```python
from build123d import *

# Parameters (mm, degrees)
F0_R     = 15
F1_DEPTH = 15
F2_R     = 15
F3_DEPTH = 10
F4_R     = 30
F4_R_2   = 15
F5_DEPTH = 10


with BuildPart() as f1:
    # F0 (on Front) → F1 (new body)
    with BuildSketch(Plane.XZ):
        with BuildLine():
            ThreePointArc((30, 15), (27.071068, 22.071068), (20, 25))
            Line((20, 25), (-20, 25))
            ThreePointArc((-20, 25), (-27.071068, 22.071068), (-30, 15))
            Line((-30, 15), (-30, -25))
            Line((-30, -25), (30, -25))
            Line((30, -25), (30, 15))
        make_face()
        with Locations((0, 5)):
            Circle(F0_R, mode=Mode.SUBTRACT)
    extrude(amount=F1_DEPTH)

    # F2 (on face) → F3 (join)
    with BuildSketch(Plane(origin=(0, 0, -25), x_dir=(1, 0, 0), z_dir=(0, 0, -1))):
        with BuildLine():
            ThreePointArc((11.14172, 62.145699), (24.842017, 73.181136), (30, 90))
            ThreePointArc((30, 90), (0, 120), (-30, 90))
            ThreePointArc((-30, 90), (-16.818864, 65.157983), (11.14172, 62.145699))
        make_face()
        with Locations((0, 90)):
            Circle(F2_R, mode=Mode.SUBTRACT)
        with BuildLine():
            ThreePointArc((11.14172, 62.145699), (-16.818864, 65.157983), (-30, 90))
            Line((-30, 90), (-30, 15))
            Line((-30, 15), (-30, 0))
            Line((-30, 0), (30, 0))
            Line((30, 0), (30, 15))
            Line((30, 15), (11.14172, 62.145699))
        make_face()
    extrude(amount=F3_DEPTH)

    # F4 (on face) → F5 (join)
    with BuildSketch(Plane(origin=(0, 0, -35), x_dir=(1, 0, 0), z_dir=(0, 0, -1))):
        with Locations((0, 90)):
            Circle(F4_R)
        with Locations((0, 90)):
            Circle(F4_R_2, mode=Mode.SUBTRACT)
    extrude(amount=F5_DEPTH)


solid = f1.part
```
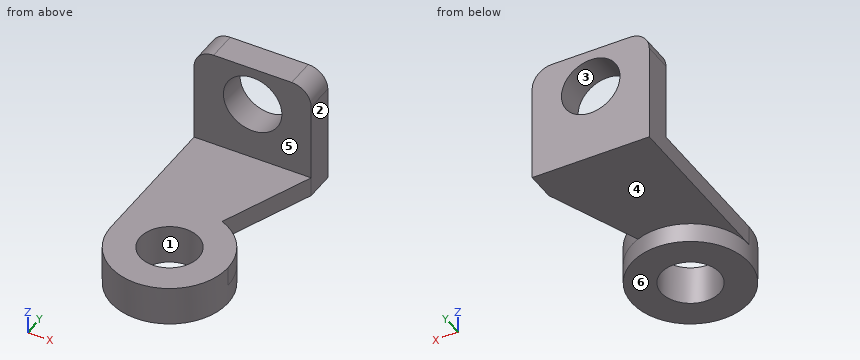
Part model, mm, in its own coordinate system. Face numbers are marked on the shaded views. A direction names the side the tool comes from. Round coordinates to 2 decimals unless told otherwise and drop trailing zeros. Order: outer loops, then holes, each group sorted by start corner. A loop starts at its lowest first (then second) coordinate and runs counter-clockwise, first axis right, second up. Notation, with made-up numbers: M 27.25,79 L 31.25,79 A19 cw 31.25,91 Z; hole C 70.25,62.25 d2. An arc over 180 degrees is marked long. Put each result on its own line as item: value. Start each with the question number.
1. Two-plate mould, pull along X, no slides. Class the marked faces 1, 2, 3 and 4: +X half, -X half, draft (parallel to the pull), parting line (faces both ways), or undercut.
2. Tool access for the marked faces 5 and 6: list every direction of +Z, -Z, +X, -X, +Y, -Y with a clear straight run to the whole face (end or side of a thin tool).
3. Slice it at B-B on z = 17. List the corners of the cut face in (x, y), then the cut area to 3 significant figures.
4. Slice it at D-D on z = -33. List the corners of the cut face in (x, y), then the cut area to 3 significant figures.
5. Drop flat-ended pins along their axis: pin 1 (10 mm diameter, centred on x = -9.5, z = 14.5, fed in from -Y); pin 2 (2 mm diameter, centred on x = 4.5, y = -34, fed in from -Z); pin 3 (5 mm diameter, centred on x = 18, y = -29, fed in from +Z). Give the stop position or say it passes through.
6. Drill centre lines: probe 1 along Z at (x, y) = (0, -4.5); probe 2 along X at (y, z) = (-90, -32); probe 3 along Z at (x, y) = (-6, -65). Where is each one in solid material? Low to high. Write a range as [from, to].
7. Slice it at C-C on y = -84. List the corners of the cut face in (x, z), then the cut area to 3 significant figures.
8. Slice it at A-A on x = 0. List the corners of the cut face in (y, z).
Findings:
1. face 1: undercut
1. face 2: +X half
1. face 3: undercut
1. face 4: draft
2. face 5: +Z, +X, -X, -Y
2. face 6: -Z, +X, -X, +Y, -Y
3. outline: M -29.8,-15 L -9,-15 L -9,0 L -29.8,0 Z; M 9,-15 L 29.8,-15 L 29.8,0 L 9,0 Z
3. area: 624 mm2
4. outline: M -30,-90 A30 ccw long 11.14,-62.15 L 30,-15 L 30,0 L -30,0 Z; hole C 0,-90 d30
4. area: 5,520 mm2
5. pin 1: y = -15
5. pin 2: z = -35
5. pin 3: z = -25
6. probe 1: [-35, -10], [20, 25]
6. probe 2: [-30, -15], [15, 30]
6. probe 3: [-45, -25]
7. outline: M -30,-35 L -29.39,-35 L -29.39,-45 L -13.75,-45 L -13.75,-25 L -30,-25 Z; M 13.75,-45 L 29.39,-45 L 29.39,-25 L 13.75,-25 Z
7. area: 632 mm2
8. outline: M -120,-45 L -105,-45 L -105,-25 L -120,-25 Z; M -75,-45 L -60,-45 L -60,-35 L 0,-35 L 0,-10 L -15,-10 L -15,-25 L -75,-25 Z; M -15,20 L 0,20 L 0,25 L -15,25 Z
